```python
from build123d import *

# Parameters (mm, degrees)
SKETCH2_R           = 4
BOSS_EXTRUDE1_DEPTH = 4
FILLET1_R           = 1


with BuildPart() as part:
    # Sketch1 → Revolve1 (revolve)
    with BuildSketch(Plane.XY):
        with BuildLine():
            ThreePointArc((0, -7), (-4.949747468, -4.949747468), (-7, 0))
            Line((-7, 0), (-10, 0))
            Line((-10, 0), (-10, -37.303915827))
            Line((-10, -37.303915827), (0, -37.303915827))
            Line((0, -37.303915827), (0, -7))
        make_face()
    revolve(axis=Axis((0, 4.024665624, 0), (0, -1, 0)))

    # Sketch2 → Boss-Extrude1 (add, symmetric)
    with BuildSketch(Plane.XY):
        with BuildLine():
            Line((-7, -51.4), (-7, -37.303915827))
            Line((-7, -37.303915827), (7, -37.303915827))
            Line((7, -37.303915827), (7, -51.4))
            ThreePointArc((7, -51.4), (0, -58.4), (-7, -51.4))
        make_face()
        with Locations((0, -51.4)):
            Circle(SKETCH2_R, mode=Mode.SUBTRACT)
    extrude(amount=BOSS_EXTRUDE1_DEPTH, both=True)

    # Fillet1
    fillet1_edges = [part.edges().sort_by_distance(p)[0] for p in [
        (0, -37.303915827, 4),
        (0, -37.303915827, -4),
        (7, -37.303915827, 0),
        (-7, -37.303915827, 0),
    ]]
    fillet(fillet1_edges, radius=FILLET1_R)


solid = part.part
```
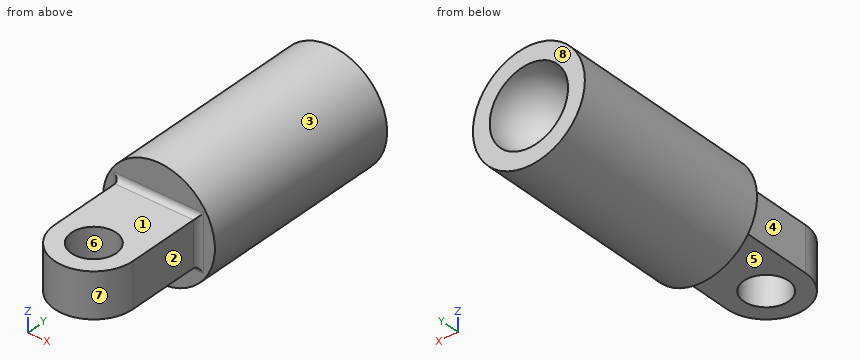
Verification items for the finished model (mm, model axes). Face numbers are marked on the shaded views. A direction names the side the tool comes from. Give positions to 0.01 mm unless a question says otherwise; leave off trailing zeros. Order: outer loops, then holes, each group sorted by start corner. A loop starts at its lowest first (then second) coordinate and runs counter-clockwise, first axis right, second up. Notation, with made-up numbers: M 39,-3.5 L 49,-3.5 A16 ccw 49,7.5 Z; hole C 48.25,47.25 d4. An arc over 180 degrees is marked long. Return JSON: item names as keys, results as strings. Group by question number.
1) Section check C-C on y = -48.5. Record the cut outline in (x, z) (3 decimals), and give its area (3 significant figures).
2) Go/stop test with flat-tipped pins: pin 1 Ø7 at (x, y) = (-3, -51.5) entering from +Z; pin 2 Ø6.5 at (y, z) = (-43, 0) entering from -X; pin 3 Ø12 at (x, z) = (-7, -7.5) entering from -Y. Record where each tip stops, or that it passes through.
3) Access from +Z, -Z, +X, -X, +Y, -Y to the whole of each face (thin tool, end or side, straight path). Record for the marked faces 1, 2, 3 and 4.
4) Section check D-D on z = 6.25. Record the cut outline in (x, y), and give its area (3 significant figures).
5) Mould release check, pull along Y, two halves, no side actions. Record for the marked faces 5, 6, 7 and 8: pulls with the +Y half, pulls with the -Y half, needs draft (parallel to the pull), parting line crosses it, or undercut.
6) Section check B-B on z = 0. Record the cut outline in (x, y), and give its area (3 significant figures).
7) Section check A-A on x = 0. Record the cut outline in (y, z), and give its area (3 significant figures).
8) Scan lines: line 1 (Y direction, x = 0, z = 0); line 2 (Z direction, x = -0.75, y = -6); line 3 (Y direction, x = 0, z = 2.5). Record each from-to range of solid material in increasing order.
Answer block:
{
 "1": {"outline": "M -7,-4 L -2.755,-4 L -2.755,4 L -7,4 Z; M 2.755,-4 L 7,-4 L 7,4 L 2.755,4 Z", "area": "67.9 mm^2"},
 "2": {"pin 1": "stops at z = 4", "pin 2": "stops at x = -7", "pin 3": "stops at y = -58.07"},
 "3": {"face 1": "+Z, +X, -X, -Y", "face 2": "+Z, -Z, +X, -Y", "face 3": "+Y, -Y", "face 4": "+Z, -Z, -X, -Y"},
 "4": {"outline": "M -7.81,-37.3 L 7.81,-37.3 L 7.81,0 L 3.15,0 A3.15 cw -3.15,0 L -7.81,0 Z", "area": "567 mm^2"},
 "5": {"face 5": "needs draft", "face 6": "undercut", "face 7": "pulls with the -Y half", "face 8": "pulls with the +Y half"},
 "6": {"outline": "M -10,-37.3 L -8,-37.3 A1 cw -7,-38.3 L -7,-51.4 A7 ccw 7,-51.4 L 7,-38.3 A1 cw 8,-37.3 L 10,-37.3 L 10,0 L 7,0 A7 cw -7,0 L -10,0 Z; hole C 0,-51.4 d8", "area": "894 mm^2"},
 "7": {"outline": "M -58.4,-4 L -55.4,-4 L -55.4,4 L -58.4,4 Z; M -47.4,-4 L -38.3,-4 A1 cw -37.3,-5 L -37.3,-10 L 0,-10 L 0,-7 A7 cw 0,7 L 0,10 L -37.3,10 L -37.3,5 A1 cw -38.3,4 L -47.4,4 Z", "area": "774 mm^2"},
 "8": {"line 1": "y = -58.4 to -55.4, -47.4 to -7", "line 2": "z = -9.97 to -3.53, 3.53 to 9.97", "line 3": "y = -58.4 to -55.4, -47.4 to -6.54"}
}
